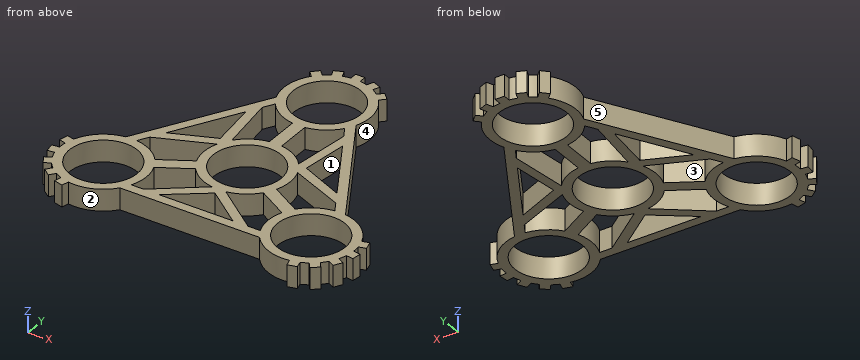
```python
from build123d import *

# Parameters (mm, degrees)
F0_R     = 11
F1_DEPTH = 7


with BuildPart() as f1:
    # F0 (on Top) → F1 (new body)
    with BuildSketch(Plane.XY):
        with BuildLine():
            Line((-12.551145, 49.429825), (-10.90317, 47.78185))
            ThreePointArc((-10.90317, 47.78185), (-13.851657, 41.032634), (-12.966522, 33.72086))
            Line((-12.966522, 33.72086), (-35.686383, -5.631093))
            ThreePointArc((-35.686383, -5.631093), (-42.461132, -8.52043), (-46.831881, -14.448503))
            Line((-46.831881, -14.448503), (-49.083057, -13.845302))
            Line((-49.083057, -13.845302), (-49.859514, -16.743079))
            Line((-49.859514, -16.743079), (-47.608338, -17.34628))
            ThreePointArc((-47.608338, -17.34628), (-47.745016, -18.584356), (-47.771108, -19.82968))
            Line((-47.771108, -19.82968), (-50.081759, -20.133883))
            Line((-50.081759, -20.133883), (-49.69018, -23.108218))
            Line((-49.69018, -23.108218), (-47.37953, -22.804015))
            ThreePointArc((-47.37953, -22.804015), (-47.032013, -24.000153), (-46.579554, -25.160667))
            Line((-46.579554, -25.160667), (-48.597904, -26.325962))
            Line((-48.597904, -26.325962), (-47.097904, -28.924038))
            Line((-47.097904, -28.924038), (-45.079554, -27.758744))
            ThreePointArc((-45.079554, -27.758744), (-44.300748, -28.730841), (-43.438621, -29.629869))
            Line((-43.438621, -29.629869), (-44.857394, -31.47885))
            Line((-44.857394, -31.47885), (-42.477334, -33.305134))
            Line((-42.477334, -33.305134), (-41.058561, -31.456153))
            ThreePointArc((-41.058561, -31.456153), (-39.967032, -32.056218), (-38.826488, -32.55689))
            Line((-38.826488, -32.55689), (-39.429689, -34.808066))
            Line((-39.429689, -34.808066), (-36.531911, -35.584523))
            Line((-36.531911, -35.584523), (-35.928711, -33.333347))
            ThreePointArc((-35.928711, -33.333347), (-28.609475, -32.512204), (-22.719861, -28.089767))
            Line((-22.719861, -28.089767), (22.719861, -28.089767))
            ThreePointArc((22.719861, -28.089767), (28.609475, -32.512204), (35.928711, -33.333347))
            Line((35.928711, -33.333347), (36.531911, -35.584523))
            Line((36.531911, -35.584523), (39.429689, -34.808066))
            Line((39.429689, -34.808066), (38.826488, -32.55689))
            ThreePointArc((38.826488, -32.55689), (39.967032, -32.056218), (41.058561, -31.456153))
            Line((41.058561, -31.456153), (42.477334, -33.305134))
            Line((42.477334, -33.305134), (44.857394, -31.47885))
            Line((44.857394, -31.47885), (43.438621, -29.629869))
            ThreePointArc((43.438621, -29.629869), (44.300748, -28.730841), (45.079554, -27.758744))
            Line((45.079554, -27.758744), (47.097904, -28.924038))
            Line((47.097904, -28.924038), (48.597904, -26.325962))
            Line((48.597904, -26.325962), (46.579554, -25.160667))
            ThreePointArc((46.579554, -25.160667), (47.032013, -24.000153), (47.37953, -22.804015))
            Line((47.37953, -22.804015), (49.69018, -23.108218))
            Line((49.69018, -23.108218), (50.081759, -20.133883))
            Line((50.081759, -20.133883), (47.771108, -19.82968))
            ThreePointArc((47.771108, -19.82968), (47.745016, -18.584356), (47.608338, -17.34628))
            Line((47.608338, -17.34628), (49.859514, -16.743079))
            Line((49.859514, -16.743079), (49.083057, -13.845302))
            Line((49.083057, -13.845302), (46.831881, -14.448503))
            ThreePointArc((46.831881, -14.448503), (42.461132, -8.52043), (35.686383, -5.631093))
            Line((35.686383, -5.631093), (12.966522, 33.72086))
            ThreePointArc((12.966522, 33.72086), (13.851657, 41.032634), (10.90317, 47.78185))
            Line((10.90317, 47.78185), (12.551145, 49.429825))
            Line((12.551145, 49.429825), (10.429825, 51.551145))
            Line((10.429825, 51.551145), (8.78185, 49.90317))
            ThreePointArc((8.78185, 49.90317), (7.777983, 50.640575), (6.712547, 51.285834))
            Line((6.712547, 51.285834), (7.604425, 53.439017))
            Line((7.604425, 53.439017), (4.832786, 54.587068))
            Line((4.832786, 54.587068), (3.940909, 52.433884))
            ThreePointArc((3.940909, 52.433884), (2.731265, 52.730994), (1.5, 52.919411))
            Line((1.5, 52.919411), (1.5, 55.25))
            Line((1.5, 55.25), (-1.5, 55.25))
            Line((-1.5, 55.25), (-1.5, 52.919411))
            ThreePointArc((-1.5, 52.919411), (-2.731265, 52.730994), (-3.940909, 52.433884))
            Line((-3.940909, 52.433884), (-4.832786, 54.587068))
            Line((-4.832786, 54.587068), (-7.604425, 53.439017))
            Line((-7.604425, 53.439017), (-6.712547, 51.285834))
            ThreePointArc((-6.712547, 51.285834), (-7.777983, 50.640575), (-8.78185, 49.90317))
            Line((-8.78185, 49.90317), (-10.429825, 51.551145))
            Line((-10.429825, 51.551145), (-12.551145, 49.429825))
        make_face()
        with Locations((-33.774991, -19.5)):
            Circle(F0_R, mode=Mode.SUBTRACT)
        Polygon((-12.018009, -25.089767), (0.191454, -16.03568), (12.018009, -25.089767), align=None, mode=Mode.SUBTRACT)
        with BuildLine():
            Line((-20.774991, -14.303848), (-11, -8.660254))
            ThreePointArc((-11, -8.660254), (-7.101984, -12.0649), (-2.233383, -13.820709))
            Line((-2.233383, -13.820709), (-16.953159, -25.089767))
            Line((-16.953159, -25.089767), (-20.939318, -25.089767))
            ThreePointArc((-20.939318, -25.089767), (-19.776615, -19.71327), (-20.774991, -14.303848))
        make_face(mode=Mode.SUBTRACT)
        with BuildLine():
            ThreePointArc((-13.085777, 4.976188), (-13.999502, -0.118049), (-13, -5.196152))
            Line((-13, -5.196152), (-22.774991, -10.839746))
            ThreePointArc((-22.774991, -10.839746), (-26.9605, -7.270416), (-32.198035, -5.589097))
            Line((-32.198035, -5.589097), (-30.204955, -2.136982))
            Line((-30.204955, -2.136982), (-13.085777, 4.976188))
        make_face(mode=Mode.SUBTRACT)
        with BuildLine():
            ThreePointArc((2.233383, -13.820709), (7.101984, -12.0649), (11, -8.660254))
            Line((11, -8.660254), (20.774991, -14.303848))
            ThreePointArc((20.774991, -14.303848), (19.776615, -19.71327), (20.939318, -25.089767))
            Line((20.939318, -25.089767), (16.953159, -25.089767))
            Line((16.953159, -25.089767), (2.233383, -13.820709))
        make_face(mode=Mode.SUBTRACT)
        with Locations((33.774991, -19.5)):
            Circle(F0_R, mode=Mode.SUBTRACT)
        with BuildLine():
            Line((22.774991, -10.839746), (13, -5.196152))
            ThreePointArc((13, -5.196152), (13.999502, -0.118049), (13.085777, 4.976188))
            Line((13.085777, 4.976188), (30.204955, -2.136982))
            Line((30.204955, -2.136982), (32.198035, -5.589097))
            ThreePointArc((32.198035, -5.589097), (26.9605, -7.270416), (22.774991, -10.839746))
        make_face(mode=Mode.SUBTRACT)
        Circle(F0_R, mode=Mode.SUBTRACT)
        Polygon((-15.719371, 22.952785), (-13.983033, 7.852036), (-27.73738, 2.136982), align=None, mode=Mode.SUBTRACT)
        with BuildLine():
            Line((-2, 25.143594), (-2, 13.856406))
            ThreePointArc((-2, 13.856406), (-6.897518, 12.182949), (-10.852394, 8.844521))
            Line((-10.852394, 8.844521), (-13.251797, 27.22675))
            Line((-13.251797, 27.22675), (-11.258717, 30.678865))
            ThreePointArc((-11.258717, 30.678865), (-7.183885, 26.983686), (-2, 25.143594))
        make_face(mode=Mode.SUBTRACT)
        with BuildLine():
            ThreePointArc((10.852394, 8.844521), (6.897518, 12.182949), (2, 13.856406))
            Line((2, 13.856406), (2, 25.143594))
            ThreePointArc((2, 25.143594), (7.183885, 26.983686), (11.258717, 30.678865))
            Line((11.258717, 30.678865), (13.251797, 27.22675))
            Line((13.251797, 27.22675), (10.852394, 8.844521))
        make_face(mode=Mode.SUBTRACT)
        Polygon((27.73738, 2.136982), (13.791579, 8.183644), (15.719371, 22.952785), align=None, mode=Mode.SUBTRACT)
        with Locations((0, 39)):
            Circle(F0_R, mode=Mode.SUBTRACT)
    extrude(amount=F1_DEPTH)


solid = f1.part
```
Here's how the part is built. I have some questions about the finished solid (model axes, mm). Face numbers are marked on the shaded views. A direction names the side the tool comes from. Coordinates: 2 decimals unless noted, no trailing zeros. Order: outer loops, then holes, each group sorted by start corner. A loop starts at its lowest first (then second) coordinate and runs counter-clockwise, first axis right, second up.
Item 1: If we section it at D-D, the plane z = 3.5: Give the number of separate pieces and of enclosed holes in the cut face, then the cut area to 3 significant figures.
Response values:
separate pieces: 1
enclosed holes: 13
area: 1,890 mm2
Item 2: If we section it at A-A, the plane y = 39: List the corners of the cut face in (x, z) for me, then the cut area to 3 significant figures.
Response values:
outline: (-14, 0) - (-11, 0) - (-11, 7) - (-14, 7) - close; (11, 0) - (14, 0) - (14, 7) - (11, 7) - close
area: 42.0 mm2
Item 3: I need wall thicknesses on probe 1 along X at (y, z) = (-26.5, 2.25); probe 2 along X at (y, z) = (51, 1.25); probe 3 along X at (y, z) = (-29.5, 5.25). Which ranges of each line are inside material? Lowest first, please.
Response values:
probe 1: x = -48.5 to -42.26, -25.29 to 25.29, 42.26 to 48.5
probe 2: x = -10.98 to -9.88, -7.21 to 7.21, 9.88 to 10.98
probe 3: x = -43.57 to -38.36, -29.19 to -23.98, 23.98 to 29.19, 38.36 to 43.57
Item 4: I'm going to push flat-ended pins straight in: pin 1 Ø3.5 at (x, z) = (-3, 4) entering from -Y; pin 2 Ø2 at (x, z) = (-19, 3) entering from +Y; pin 3 Ø2 at (y, z) = (20, 2.5) entering from +X. Where does each tip first touch, or does it pass through?
Response values:
pin 1: stops at y = -28.09
pin 2: stops at y = 25
pin 3: stops at x = 21.47
Item 5: If we section it at B-B, the plane y = -12.5: List the corners of the cut face in (x, z) for me.
Response values:
outline: (-45.9, 0) - (-42.26, 0) - (-42.26, 7) - (-45.9, 7) - close; (-25.29, 0) - (-17.65, 0) - (-17.65, 7) - (-25.29, 7) - close; (-6.3, 0) - (6.3, 0) - (6.3, 7) - (-6.3, 7) - close; (17.65, 0) - (25.29, 0) - (25.29, 7) - (17.65, 7) - close; (42.26, 0) - (45.9, 0) - (45.9, 7) - (42.26, 7) - close
Item 6: Thinking about a two-plate mould opening in X: for the marked faces 3, 4 and 5, which applies, pulls with the +X half, pulls with the -X half, needs draft (parallel to the pull), parting line crosses it, or undercut?
Response values:
face 3: undercut
face 4: pulls with the +X half
face 5: pulls with the -X half
Item 7: Which directions (+Z, -Z, +X, -X, +Y, -Y) give clear straight access to the entire face, cutting with the end or side of a thin tool? Please do the marked faces 1 and 2.
Response values:
face 1: +Z, -Z
face 2: +Z, -Z, -Y
Item 8: If we section it at C-C, the plane y = 0: List the corners of the cut face in (x, z) for me, then the cut area to 3 significant figures.
Response values:
outline: (-32.44, 0) - (-25.06, 0) - (-25.06, 7) - (-32.44, 7) - close; (-14, 0) - (-11, 0) - (-11, 7) - (-14, 7) - close; (11, 0) - (14, 0) - (14, 7) - (11, 7) - close; (25.06, 0) - (32.44, 0) - (32.44, 7) - (25.06, 7) - close
area: 145 mm2
